Input: part model. Units: mm. Frame: model coordinates. Coordinates: 2 decimals unless noted, no trailing zeros. Loops run counter-clockwise (first coordinate to the right, second up) from the corner with the lowest first, then second, coordinate; pieces in that order, holes last. Notation, with made-up numbers: (68.25, 47.25) -> (83.25, 47.25) arc R18 ccw to (83.25, 60.25) -> close; hole circle Ø9 at (19.5, -7.5). An arc over 180 degrees is marked (long way). Answer as a JSON object with one key per item and string values.
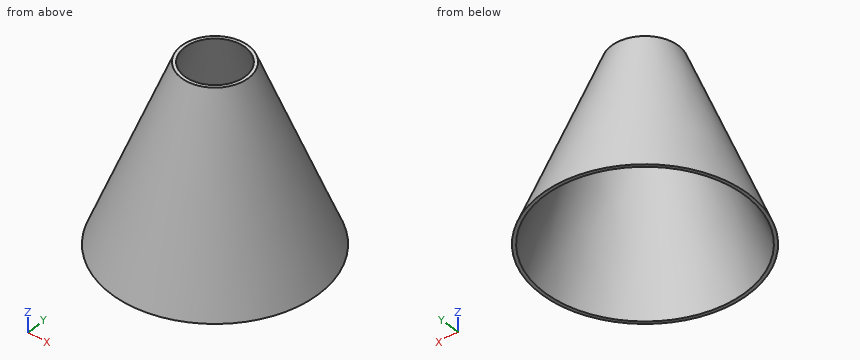
from build123d import *

# Parameters (mm, degrees)
CYLINDER044_R     = 8
CYLINDER044_DEPTH = 3


with BuildPart() as cylinder044:
    # Cylinder044 → Cylinder044 (new body)
    with BuildSketch(Plane.XY.offset(123)):
        Circle(CYLINDER044_R)
    extrude(amount=CYLINDER044_DEPTH)


with BuildPart() as cone001:
    # Cone002 → Cone002 (revolve)
    with BuildSketch(Plane(origin=(0, 0, 75), x_dir=(1, 0, 0), z_dir=(0, -1, 0))):
        Polygon((0, 0), (21.5, 0), (5.3, 41), (0, 41), align=None)
    revolve(axis=Axis((0, 0, 75), (0, 0, 1)))


with BuildPart() as conical_section:
    # Cone001 → Cone001 (revolve)
    with BuildSketch(Plane(origin=(0, 0, 75), x_dir=(1, 0, 0), z_dir=(0, -1, 0))):
        Polygon((0, 0), (22.2, 0), (6, 41), (0, 41), align=None)
    revolve(axis=Axis((0, 0, 75), (0, 0, 1)))

    # Cut003: cut Cone001
    add(cone001.part, mode=Mode.SUBTRACT)


with BuildPart() as conical_section_1:
    # Cut003 placement: moved
    add(conical_section.part.moved(Location((0, 0, 10))))

    # Cut038: cut Cylinder044
    add(cylinder044.part, mode=Mode.SUBTRACT)


solid = conical_section_1.part
1. Section query C-C (z = 118). Return loops of the section in (x, y).
Reply:
{"outline": "circle Ø18.32 at (0, 0); hole circle Ø16.92 at (0, 0)"}
2. Section query D-D (z = 113.5). Return loops of the section in (x, y).
Reply:
{"outline": "circle Ø21.88 at (0, 0); hole circle Ø20.48 at (0, 0)"}
3. Section query A-A (y = 0). Return loops of the section in (x, z), plus the area to 3 significant figures.
Reply:
{"outline": "(-22.2, 85) -> (-21.5, 85) -> (-6.49, 123) -> (-7.19, 123) -> close; (6.49, 123) -> (21.5, 85) -> (22.2, 85) -> (7.19, 123) -> close", "area": "53.2 mm2"}
4. Pin query (flat end, axial travel): P1, Ø2, axis at x = 16, y = 15.5, coming from the -Z side; P2, Ø10, axis at x = -6, z = 118, coming from the +Y side; P3, Ø8, axis at y = 9, z = 108.5, coming from the +X side; P4, Ø2, axis at x = -3.5, z = 110, coming from the +Y side. Return the tip coordinate at first contact, or that it passes through.
Reply:
{"P1": "stops at z = 85", "P2": "stops at y = 10.31", "P3": "stops at x = 12.61", "P4": "stops at y = 12.3"}
5. Line query: line 1 along X through (y, z) = (8.5, 107); line 2 along X through (y, z) = (-10, 90); line 3 along Y through (x, z) = (13.5, 102). Output: solid intervals per line, ascending.
Reply:
{"line 1": "x = -10.5 to -9.58, 9.58 to 10.5", "line 2": "x = -17.58 to -16.77, 16.77 to 17.58", "line 3": "y = -7.58 to -6.02, 6.02 to 7.58"}
